Geometry: final body of the model. Coordinates: model frame, mm. A direction names the side the tool comes from. Give positions to 0.01 mm unless a question says otherwise; leave off trailing zeros. Write each loop counter-clockwise with the first axis right and the second up, starting at its lowest first coordinate (ties: lowest second). Pieces come first, ordered by that corner, then holes.
Q1. Reachability of faces 4 (the flat face through (238, -231, -400.415)), 5 (the cylindrical face through (3.819, -308.605, -587.317)), 6 (the cylindrical face through (3.82, -58.38, -168.94)), 7 (the flat face through (238, -6, -711.816)), 8 (the flat face through (238, -31.759, -587)) from +Z, -Z, +X, -X, +Y, -Y: full face, straight path, thin tool, end or side. Return the list, or none.
Q2. Line query: line 1 (Z direction, x = 259.5, y = -23.5); line 2 (Z direction, x = 112.5, y = -346.5); line 3 (Y direction, x = 418, z = -411.5). Output: solid intervals per line, ascending.
Q3. Section A-A (x = 77.5). Return the cut outline in (y, z).
Q4. Mould query, pull axis Y, two halves, no side actions, for faces 1 (the flat face through (0, -60, -379)), 2 (the flat face through (238, -385.953, -557)), 3 (the cylindrical face through (478.781, -308.605, -587.317)). Classes: +Y half, -Y half, draft (parallel to the pull), parting line (faces both ways), or undercut.
Q5. Pin query (flat end, axial travel): pin 1 Ø6 at (x, y) = (146.5, -177) entering from -Z; pin 2 Ø1 at (x, y) = (433, -227) entering from +Z; pin 3 Ø4 at (x, y) = (264, -269.5) entering from -Z. Return the tip coordinate at first contact, or that it passes through.
Q6. Section B-B (y = -244.5). Return the cut outline in (x, z), plus the area to 3 significant figures.
from build123d import *

# Parameters (mm, degrees)
F1_DEPTH = 482.6
F2_R     = 12.7


with BuildPart() as f1:
    # F0 (on Right) → F1 (new body)
    with BuildSketch(Plane.YZ):
        Polygon((33.734092, 69.37997), (-42.465908, 69.37997), (-80.995351, -400.415391), (-385.953367, -400.415391), (-385.953367, -718.258917), (-336.558729, -718.258917), (-272.130996, -451.957613), (-31.758729, -451.957613), (-31.758729, -711.816192), (33.734092, -711.816192), align=None)
    extrude(amount=F1_DEPTH)

    # F2
    f2_edges = [f1.edges().sort_by_distance(p)[0] for p in [
        (241.3, -385.953367, -400.415391),
        (241.3, -385.953367, -718.258917),
        (0, -385.953367, -559.337154),
        (482.6, -385.953367, -559.337154),
        (241.3, -80.995351, -400.415391),
        (0, -233.474359, -400.415391),
        (482.6, -233.474359, -400.415391),
        (482.6, -4.365908, 69.37997),
        (482.6, -61.730629, -165.51771),
        (482.6, -361.256048, -718.258917),
        (482.6, -304.344863, -585.108265),
        (482.6, -151.944863, -451.957613),
        (482.6, -31.758729, -581.886902),
        (482.6, 0.987682, -711.816192),
        (482.6, 33.734092, -321.218111),
        (241.3, -42.465908, 69.37997),
        (0, -61.730629, -165.51771),
        (241.3, 33.734092, 69.37997),
        (0, -4.365908, 69.37997),
        (241.3, 33.734092, -711.816192),
        (0, 33.734092, -321.218111),
        (0, -361.256048, -718.258917),
        (0, -304.344863, -585.108265),
        (0, -151.944863, -451.957613),
        (0, -31.758729, -581.886902),
        (0, 0.987682, -711.816192),
        (241.3, -272.130996, -451.957613),
        (241.3, -31.758729, -451.957613),
    ]]
    fillet(f2_edges, radius=F2_R)


solid = f1.part
Computed:
1. face 4: +Z, +X, -X, -Y
1. face 5: -Z, -X
1. face 6: +Z, -X, -Y
1. face 7: -Z, +X, -X, +Y
1. face 8: -Z, +X, -X
2. line 1: z = -711.82 to 69.38
2. line 2: z = -718.26 to -400.42
2. line 3: y = -385.85 to 33.73
3. outline: (-385.95, -705.56) arc R12.7 ccw to (-373.25, -718.26) - (-336.56, -718.26) - (-274.48, -461.67) arc R12.7 cw to (-262.14, -451.96) - (-44.46, -451.96) arc R12.7 cw to (-31.76, -464.66) - (-31.76, -711.82) - (21.03, -711.82) arc R12.7 ccw to (33.73, -699.12) - (33.73, 56.68) arc R12.7 ccw to (21.03, 69.38) - (-30.76, 69.38) arc R12.7 ccw to (-43.42, 57.72) - (-80.04, -388.75) arc R12.7 cw to (-92.7, -400.42) - (-373.25, -400.42) arc R12.7 ccw to (-385.95, -413.12) - close
4. face 1: draft
4. face 2: -Y half
4. face 3: undercut
5. pin 1: stops at z = -451.96
5. pin 2: stops at z = -400.42
5. pin 3: stops at z = -456.08
6. outline: (0, -439.26) arc R12.7 ccw to (12.7, -451.96) - (469.9, -451.96) arc R12.7 ccw to (482.6, -439.26) - (482.6, -413.12) arc R12.7 ccw to (469.9, -400.42) - (12.7, -400.42) arc R12.7 ccw to (0, -413.12) - close
6. area: 24,700 mm2
